Could you check a few things on this drawing? It's one solid part, dimensions in mm from its lowest x, y, z. A direction names the side the tool comes from. Coordinates: 2 decimals unless noted, no trailing zeros. Order: outer loops, then holes, each group sorted by start corner. A loop starts at its lowest first (then second) coordinate and runs counter-clockwise, first axis right, second up.
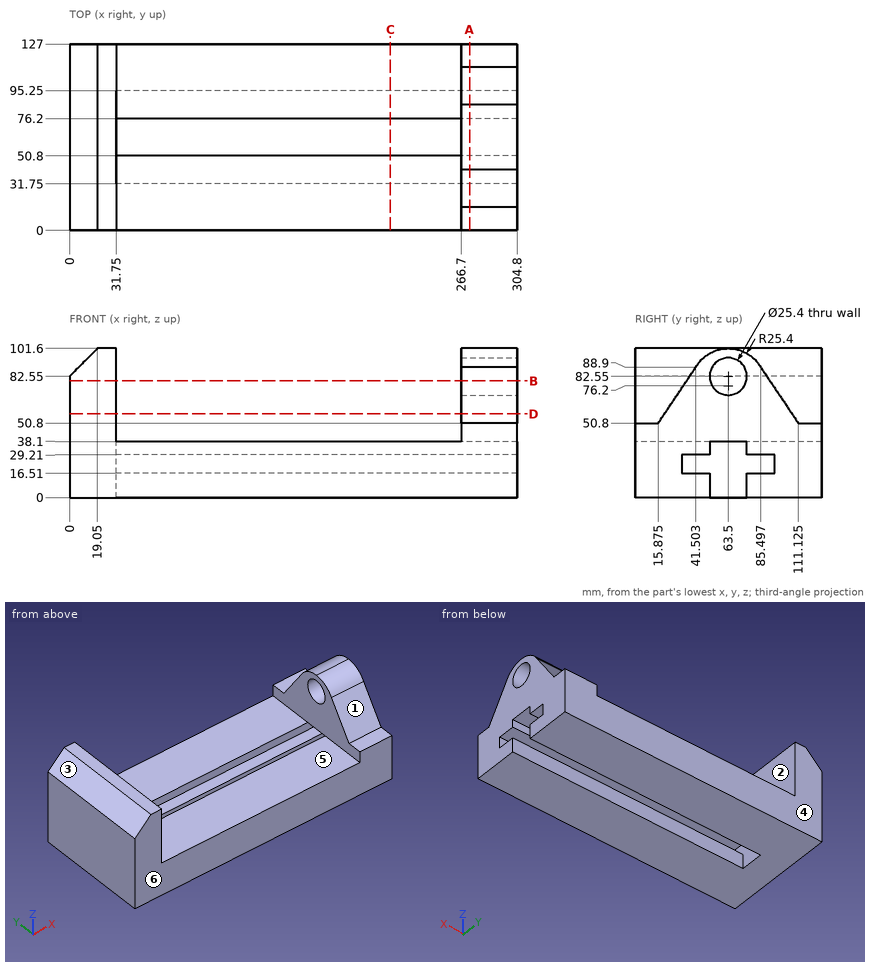
1. Imagine slicing it at D-D on z = 57. Please give me the cut outline in (x, y), then the cut area to 3 significant figures.
Completed:
outline: (0, 0) - (31.75, 0) - (31.75, 127) - (0, 127) - close; (266.7, 20.05) - (304.8, 20.05) - (304.8, 106.95) - (266.7, 106.95) - close
area: 7,340 mm2
2. Imagine slicing it at A-A on x = 272.5. Please give me the cut outline in (y, z) (3 decimals).
Completed:
outline: (0, 0) - (50.8, 0) - (50.8, 16.51) - (31.75, 16.51) - (31.75, 29.21) - (50.8, 29.21) - (50.8, 38.1) - (76.2, 38.1) - (76.2, 29.21) - (95.25, 29.21) - (95.25, 16.51) - (76.2, 16.51) - (76.2, 0) - (127, 0) - (127, 50.8) - (111.125, 50.8) - (85.497, 88.9) arc R25.4 ccw to (63.5, 101.6) arc R25.4 ccw to (41.503, 88.9) - (15.875, 50.8) - (0, 50.8) - close; hole circle Ø25.4 at (63.5, 82.55)
3. I'm going to push flat-ended pins straight in: pin 1 (8 mm diameter, centred on y = 74.5, z = 78, fed in from +X); pin 2 (15 mm diameter, centred on x = 174.5, y = 88, fed in from +Z); pin 3 (17.5 mm diameter, centred on x = 279.5, y = 11, fed in from +Z); pin 4 (3 mm diameter, centred on y = 114, z = 76.5, fed in from +X). Where does each tip first touch, or does it pass through?
Completed:
pin 1: stops at x = 304.8
pin 2: stops at z = 38.1
pin 3: stops at z = 56.56
pin 4: stops at x = 31.75
4. On a 3-axis mill with a long thin cutter (end or side, diameter ignored), from which of +Z, -Z, +X, -X, +Y, -Y can I reach the whole of each face in a straight line? I mean the marked faces 5 and 6. Say none if no direction works.
Completed:
face 5: +Z, +Y, -Y
face 6: +Z, -Z, +X, -X, -Y
5. Thinking about a two-plate mould opening in Y: for the marked faces 1, 2, 3 and 4, which applies, pulls with the +Y half, pulls with the -Y half, needs draft (parallel to the pull), parting line crosses it, or undercut?
Completed:
face 1: pulls with the -Y half
face 2: undercut
face 3: needs draft
face 4: pulls with the +Y half
6. Imagine slicing it at C-C on x = 218.5. Please give me the cut outline in (y, z).
Completed:
outline: (0, 0) - (50.8, 0) - (50.8, 16.51) - (31.75, 16.51) - (31.75, 29.21) - (50.8, 29.21) - (50.8, 38.1) - (0, 38.1) - close; (76.2, 0) - (127, 0) - (127, 38.1) - (76.2, 38.1) - (76.2, 29.21) - (95.25, 29.21) - (95.25, 16.51) - (76.2, 16.51) - close
7. Imagine slicing it at B-B on z = 79.5. Please give me the cut outline in (x, y), then the cut area to 3 significant figures.
Completed:
outline: (0, 0) - (31.75, 0) - (31.75, 127) - (0, 127) - close; (266.7, 35.18) - (304.8, 35.18) - (304.8, 51.17) - (266.7, 51.17) - close; (266.7, 75.83) - (304.8, 75.83) - (304.8, 91.82) - (266.7, 91.82) - close
area: 5,250 mm2
8. Please list where these lines run through material, in increasing order: probe 1 along X at (y, z) = (81.5, 82); probe 2 along Z at (x, y) = (296, 63) (3 decimals); probe 3 along Z at (x, y) = (56, 78).
Completed:
probe 1: x = 0 to 31.75, 266.7 to 304.8
probe 2: z = 38.1 to 69.86, 95.24 to 101.595
probe 3: z = 0 to 16.51, 29.21 to 38.1
